Design review of the part built by this model. Coordinates are the model's own, in mm. Face numbers are marked on the shaded views. A direction names the side the tool comes from. Give positions to 0.01 mm unless a question says otherwise; leave off trailing zeros. Write each loop counter-clockwise with the first axis right and the second up, starting at its lowest first coordinate (ties: lowest second). Pieces come first, ordered by that corner, then holes. Notation, with made-up numbers: M -12,-25 L 12,-25 A12 ccw 12,-8 Z; hole C -15.75,-22 d3. An arc over 180 degrees is marked long. Answer in a Markdown table with one row per item.
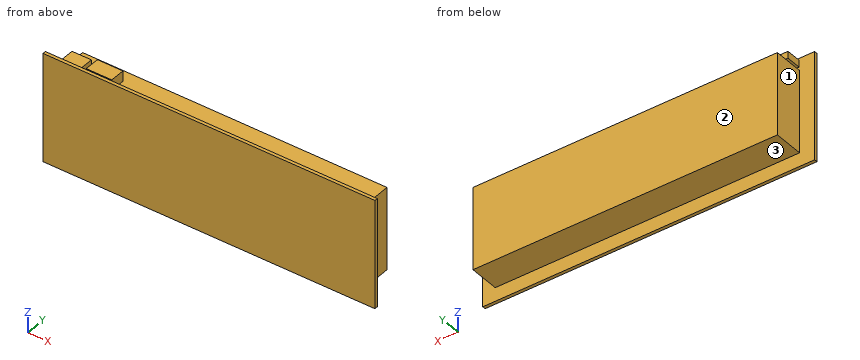
```python
from build123d import *

# Parameters (mm, degrees)
SKETCH1_W           = 265.36
SKETCH1_H           = 86.74
BOSS_EXTRUDE1_DEPTH = 2.56
SKETCH2_W           = 243.36
SKETCH2_H           = 65.94
BOSS_EXTRUDE2_DEPTH = 24
SKETCH3_W           = 15.5
SKETCH3_H           = 5.5
SKETCH3_W_2         = 20.4
SKETCH3_H_2         = 8.3
BOSS_EXTRUDE3_DEPTH = 12


with BuildPart() as part:
    # Sketch1 → Boss-Extrude1 (new body)
    with BuildSketch(Plane(origin=(0, 0, 0), x_dir=(1, 0, 0), z_dir=(0, 1, 0))):
        with Locations((132.68, 43.37)):
            Rectangle(SKETCH1_W, SKETCH1_H)
    extrude(amount=BOSS_EXTRUDE1_DEPTH)

    # Sketch2 → Boss-Extrude2 (add)
    with BuildSketch(Plane(origin=(0, 2.56, 0), x_dir=(1, 0, 0), z_dir=(0, 1, 0))):
        with Locations((133.68, 42.87)):
            Rectangle(SKETCH2_W, SKETCH2_H)
    extrude(amount=BOSS_EXTRUDE2_DEPTH)

    # Sketch3 → Boss-Extrude3 (add)
    with BuildSketch(Plane(origin=(0, 2.56, 0), x_dir=(1, 0, 0), z_dir=(0, 1, 0))):
        with Locations((20.15, 4.25)):
            Rectangle(SKETCH3_W, SKETCH3_H)
        with Locations((42.9, 3.35)):
            Rectangle(SKETCH3_W_2, SKETCH3_H_2)
    extrude(amount=BOSS_EXTRUDE3_DEPTH)


solid = part.part
```
1) Add section A-A (y = 5). Write out the cut boundary in (x, z).
Geometry says:
| item | result |
|---|---|
| outline | M 12,-75.84 L 255.36,-75.84 L 255.36,-9.9 L 12,-9.9 Z; M 12.4,-7 L 27.9,-7 L 27.9,-1.5 L 12.4,-1.5 Z; M 32.7,-7.5 L 53.1,-7.5 L 53.1,0.8 L 32.7,0.8 Z |
2) To check wall thickness, follow probe 1 along X at (y, z) = (23, -41); probe 2 along Z at (x, y) = (162, 17.25); probe 3 along Y at (x, z) = (138, -78). State the ranges of each line that lie inside material, in increasing order. Write a range as [from, to].
Geometry says:
| item | result |
|---|---|
| probe 1 | [12, 255.36] |
| probe 2 | [-75.84, -9.9] |
| probe 3 | [0, 2.56] |
3) Add section C-C (z = -64). Write out the cut boundary in (x, y).
Geometry says:
| item | result |
|---|---|
| outline | M 0,0 L 265.36,0 L 265.36,2.56 L 255.36,2.56 L 255.36,26.56 L 12,26.56 L 12,2.56 L 0,2.56 Z |
4) For the marked faces 1, 2 and 3, list the 3-axis set-ups (+Z, -Z, +X, -X, +Y, -Y) from which the entire face can be reached by the end or side of a thin tool; tool diameter is ignored.
Geometry says:
| item | result |
|---|---|
| face 1 | +Z, -Z, -X, +Y |
| face 2 | +Z, -Z, +X, -X, +Y |
| face 3 | -Z, +X, -X, +Y |
5) Add section B-B (x = 43.5). Write out the cut boundary in (y, z).
Geometry says:
| item | result |
|---|---|
| outline | M 0,-86.74 L 2.56,-86.74 L 2.56,-75.84 L 26.56,-75.84 L 26.56,-9.9 L 2.56,-9.9 L 2.56,-7.5 L 14.56,-7.5 L 14.56,0.8 L 2.56,0.8 L 2.56,0 L 0,0 Z |
6) Insertion check: P1, Ø3.5, axis at x = 47, y = 6.5, coming from the -Z side; P2, Ø7, axis at y = 15.5, z = -36, coming from the +X side; P3, Ø6.5, axis at y = 11, z = -2, coming from the -X side. Each pin has a flat end and moves straight along its axis. Give the tip position at first contact, or say it passes through.
Geometry says:
| item | result |
|---|---|
| P1 | z = -75.84 |
| P2 | x = 255.36 |
| P3 | x = 12.4 |
7) Add section D-D (x = 123). Write out the cut boundary in (y, z).
Geometry says:
| item | result |
|---|---|
| outline | M 0,-86.74 L 2.56,-86.74 L 2.56,-75.84 L 26.56,-75.84 L 26.56,-9.9 L 2.56,-9.9 L 2.56,0 L 0,0 Z |
